Geometry: final body of the model. Coordinates: model frame, mm. A direction names the side the tool comes from. Coordinates: 2 decimals unless noted, no trailing zeros. Order: outer loops, then holes, each group sorted by start corner. A loop starts at its lowest first (then second) coordinate and runs counter-clockwise, first axis right, second up. Notation, with made-up numbers: (62, 17.5) -> (104, 17.5) arc R18 cw to (104, 34.5) -> close; hole circle Ø10 at (-7.75, 4.25). An arc over 180 degrees is marked (long way). Use one line per item in the form item = value.
```python
from build123d import *

# Parameters (mm, degrees)
BOSS_EXTRUDE1_DEPTH = 200
CUT_EXTRUDE1_REACH  = 214.512
SKETCH2_R           = 4


with BuildPart() as part:
    # Sketch1 → Boss-Extrude1 (new, symmetric)
    with BuildSketch(Plane(origin=(0, 0, 0), x_dir=(0, 0, -1), z_dir=(1, 0, 0))):
        Polygon((0, 50.8), (0, 0), (-50.8, 0), (-50.8, 6.35), (-6.35, 6.35), (-6.35, 50.8), align=None)
    extrude(amount=BOSS_EXTRUDE1_DEPTH, both=True)

    # Sketch2 → Cut-Extrude1 (cut, up to next)
    with BuildSketch(Plane.XZ, mode=Mode.PRIVATE) as cut_extrude1_sk1:
        with Locations(Location((-185, 25.4, 0), (0, 0, 270))):
            Circle(SKETCH2_R)
    cut_extrude1_tool1 = extrude(cut_extrude1_sk1.sketch, amount=-CUT_EXTRUDE1_REACH, mode=Mode.PRIVATE) & part.part
    # Sketch2 → Cut-Extrude1 (cut, up to next)
    with BuildSketch(Plane.XZ, mode=Mode.PRIVATE) as cut_extrude1_sk2:
        with Locations(Location((185, 25.4, 0), (0, 0, 270))):
            Circle(SKETCH2_R)
    cut_extrude1_tool2 = extrude(cut_extrude1_sk2.sketch, amount=-CUT_EXTRUDE1_REACH, mode=Mode.PRIVATE) & part.part
    cut_extrude1_1 = cut_extrude1_tool1.solids().sort_by_distance((-185, 0, 25.4))[0]
    add(cut_extrude1_1, mode=Mode.SUBTRACT)
    cut_extrude1_2 = cut_extrude1_tool2.solids().sort_by_distance((185, 0, 25.4))[0]
    add(cut_extrude1_2, mode=Mode.SUBTRACT)
    cut_extrude1 = cut_extrude1_1 + cut_extrude1_2  # Cut-Extrude1 as one shape, for the pattern or mirror that repeats it

    # Mirror1: Cut-Extrude1 across plane
    add(cut_extrude1.mirror(Plane(origin=(0, 0, 0), x_dir=(0, 0.7071067811865471, 0.7071067811865479), z_dir=(0, -0.7071067811865479, 0.7071067811865471))), mode=Mode.SUBTRACT)


solid = part.part
```
1) Access query for faces 1 (the flat face through (3, 0, 25)), 2 (the flat face through (3, 28, 6.35)). Directions: +Z, -Z, +X, -X, +Y, -Y. A direction counts if a zero-diameter tool reaches every point of the face in a straight line with its end or side. Return the directions, or none.
Results found:
face_1 = +Z, -Z, +X, -X, -Y
face_2 = +Z, +X, -X, +Y
2) Material intervals for probe 1 along X at (y, z) = (4, 25); probe 2 along Y at (x, z) = (185, 2.75); probe 3 along Z at (x, y) = (-74.5, 40), sorted ascending. Write a range as from..to.
Results found:
probe_1 = -200..-188.98, -181.02..181.02, 188.98..200
probe_2 = 0..21.4, 29.4..50.8
probe_3 = 0..6.35
3) Pull-direction query (X, two-part tool) for faces 3 (the flat face through (3, 6.35, 29)), 4 (the cylindrical face through (-181.034, 3.131, 25.921)), 5 (the flat face through (-200, 5, 14)), 6 (the cylindrical face through (188.966, 3.131, 25.921)); classes: released by +X, released by -X, zero draft, split by the parting line, or undercut.
Results found:
face_3 = zero draft
face_4 = undercut
face_5 = released by -X
face_6 = undercut
4) Section B-B, the plane z = 25.4. Output: boundary loops of the cut face in (x, y), and give its area (3 significant figures).
Results found:
outline = (-200, 0) -> (-189, 0) -> (-189, 6.35) -> (-200, 6.35) -> close; (-181, 0) -> (181, 0) -> (181, 6.35) -> (-181, 6.35) -> close; (189, 0) -> (200, 0) -> (200, 6.35) -> (189, 6.35) -> close
area = 2,440 mm2
5) Section D-D, the plane x = 129.5. Output: boundary loops of the cut face in (y, z).
Results found:
outline = (0, 0) -> (50.8, 0) -> (50.8, 6.35) -> (6.35, 6.35) -> (6.35, 50.8) -> (0, 50.8) -> close
6) Contact query for flat-ended pins moving along their axis: P1, Ø4, axis at x = -4, z = 19, coming from the +Y side; P2, Ø10.5, axis at x = 185, y = 25.4, coming from the +Z side; P3, Ø5, axis at x = 185, z = 25.4, coming from the -Y side. Output: stop coordinate, or through.
Results found:
P1 = 6.35
P2 = 6.35
P3 = through
7) Section A-A, the plane x = 185. Output: boundary loops of the cut face in (y, z).
Results found:
outline = (0, 0) -> (21.4, 0) -> (21.4, 6.35) -> (6.35, 6.35) -> (6.35, 21.4) -> (0, 21.4) -> close; (0, 29.4) -> (6.35, 29.4) -> (6.35, 50.8) -> (0, 50.8) -> close; (29.4, 0) -> (50.8, 0) -> (50.8, 6.35) -> (29.4, 6.35) -> close
